Part print with two shaded views. Sizes in mm from the minimum x, y, z corner. A direction names the side the tool comes from. Give positions to 0.01 mm unless a question says otherwise; leave off trailing zeros. Write each loop counter-clockwise with the first axis right and the second up, starting at its lowest first coordinate (ties: lowest second). Pieces come first, ordered by that corner, then holes.
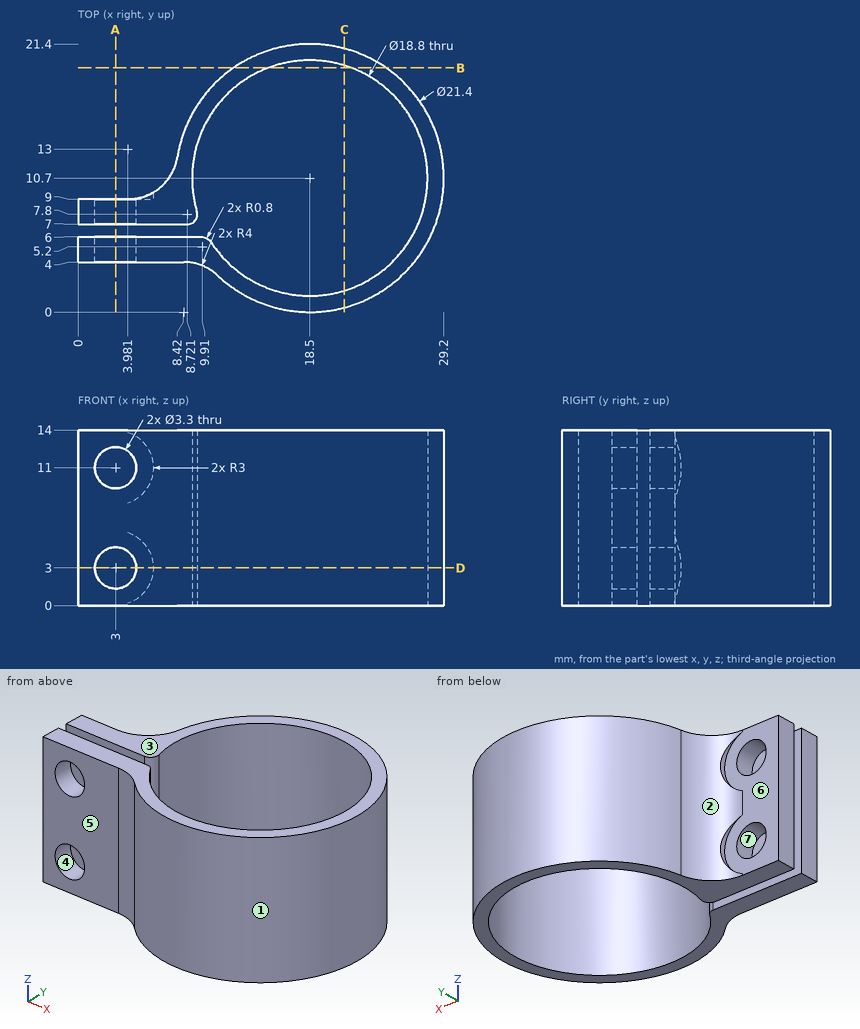
1) Saw through at B-B, the plane y = 19.5. Write the cut outline in (x, z) (1 decimal).
Answers follow:
outline: (12.4, 0) - (15.2, 0) - (15.2, 14) - (12.4, 14) - close; (21.8, 0) - (24.6, 0) - (24.6, 14) - (21.8, 14) - close
2) Saw through at A-A, the plane x = 3. Write the cut outline in (y, z), then the cut area to 3 significant figures.
Answers follow:
outline: (4, 0) - (6, 0) - (6, 1.35) - (4, 1.35) - close; (4, 4.65) - (6, 4.65) - (6, 9.35) - (4, 9.35) - close; (4, 12.65) - (6, 12.65) - (6, 14) - (4, 14) - close; (7, 0) - (9, 0) - (9, 1.35) - (7, 1.35) - close; (7, 4.65) - (9, 4.65) - (9, 9.35) - (7, 9.35) - close; (7, 12.65) - (9, 12.65) - (9, 14) - (7, 14) - close
area: 29.6 mm2
3) Saw through at D-D, the plane z = 3. Count the separate pieces of the cut face and the enclosed holes in it.
Answers follow:
separate pieces: 3
enclosed holes: 0
4) Pin check, flat tips, straight feed: pin 1 Ø2 at (y, z) = (19, 9) entering from -X; pin 2 Ø4.5 at (x, z) = (3, 3) entering from +Y; pin 3 Ø5 at (x, z) = (24, 10.5) entering from +Y; pin 4 Ø3 at (x, z) = (3, 3) entering from -Y. Stop position of each tip, or through.
Answers follow:
pin 1: stops at x = 10.68
pin 2: stops at y = 9
pin 3: stops at y = 20.97
pin 4: passes through
5) Two-plate mould, pull along X, no slides. Class the marked faces 1, 2, 3 and 4: +X half, -X half, draft (parallel to the pull), parting line (faces both ways), or undercut.
Answers follow:
face 1: parting line
face 2: -X half
face 3: draft
face 4: undercut
6) 3-axis set-ups, long thin cutter, end or side, ignore diameter. For the marked faces 5, 6 and 7: which of +Z, -Z, +X, -X, +Y, -Y reach the whole face in a straight line?
Answers follow:
face 5: +Z, -Z, -X, -Y
face 6: -X, +Y
face 7: +Y, -Y
7) Wall check: L1, parallel to Z at x = 3, y = 5.45; L2, parallel to Y at x = 2, z = 8.5; L3, parallel to X at y = 14, z = 2. Give the ranges that are in metal, low to high.
Answers follow:
L1: z = 0 to 1.35, 4.65 to 9.35, 12.65 to 14
L2: y = 4 to 6, 7 to 9
L3: x = 8.32 to 9.7, 27.3 to 28.68
8) Saw through at C-C, the plane x = 21.25. Write the cut outline in (y, z).
Answers follow:
outline: (0.36, 0) - (1.71, 0) - (1.71, 14) - (0.36, 14) - close; (19.69, 0) - (21.04, 0) - (21.04, 14) - (19.69, 14) - close
